Verification items for the finished model (mm, model axes). Face numbers are marked on the shaded views. A direction names the side the tool comes from. Round coordinates to 2 decimals unless told otherwise and drop trailing zeros. Write each loop counter-clockwise with the first axis right and the second up, starting at its lowest first coordinate (ties: lowest second). Pieces come first, ordered by that corner, then holes.
from build123d import *

# Parameters (mm, degrees)
F0_W     = 50.8894138038
F0_H     = 50.8894175291
F1_DEPTH = 50.8
F2_W     = 25.4447069019
F2_H     = 25.3969691694
F3_DEPTH = 50.8
F5_DEPTH = 25.4


with BuildPart() as f1:
    # F0 (on Front) → F1 (new body)
    with BuildSketch(Plane.XZ):
        with Locations((25.4447069019, 25.4447087646)):
            Rectangle(F0_W, F0_H)
    extrude(amount=F1_DEPTH)

    # F2 (on face) → F3 (cut)
    with BuildSketch(Plane.XZ.offset(50.8)):
        with Locations((38.1670603529, 38.1909329444)):
            Rectangle(F2_W, F2_H)
    extrude(amount=-F3_DEPTH, mode=Mode.SUBTRACT)

    # F4 (on face) → F5 (join)
    with BuildSketch(Plane.YZ.offset(25.4447069019)):
        Polygon((0, 50.8894175291), (-25.4, 50.8894175291), (-25.4, 25.4924483597), (0, 25.4924483597), (0, 29.243901372), (0, 43.372977525), align=None)
    extrude(amount=F5_DEPTH)


solid = f1.part
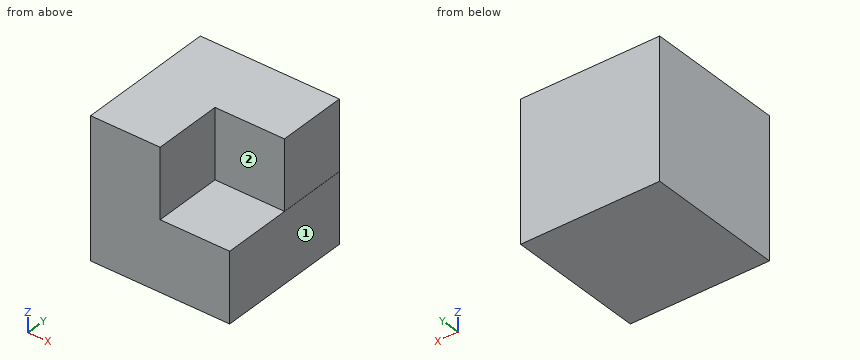
Q1. Sectioned sample at B-B (y = -29). Enter the section's corners in (x, z), plus the area to 3 significant figures.
Recorded:
outline: (0, 0) - (50.89, 0) - (50.89, 25.49) - (25.44, 25.49) - (25.44, 50.89) - (0, 50.89) - close
area: 1,940 mm2
Q2. Material ranges on line 1 along Y through (x, z) = (34, 27); line 2 along Z through (x, y) = (47, -35.5); line 3 along X through (y, z) = (-45, 30), recorded low to high.
Recorded:
line 1: y = -25.4 to 0
line 2: z = 0 to 25.49
line 3: x = 0 to 25.44
Q3. Depth check by flat-ended pin: P1, Ø3, axis at x = 31.5, y = -42.5, coming from the +Z side; P2, Ø7.5, axis at y = -41.5, z = 33, coming from the +X side; P3, Ø7.5, axis at y = -14.5, z = 32.5, coming from the +X side. Enter the tip coordinate at first touch or a pass-through.
Recorded:
P1: stops at z = 25.49
P2: stops at x = 25.44
P3: stops at x = 50.84
Q4. Sectioned sample at A-A (z = 47.5). Enter the section's corners in (x, y).
Recorded:
outline: (0, -50.8) - (25.44, -50.8) - (25.44, -25.4) - (50.84, -25.4) - (50.84, 0) - (0, 0) - close
Q5. Tool access check on the marked faces 1 and 2. Record the directions out of +Z, -Z, +X, -X, +Y, -Y that give a thin tool (end or side, any length) a straight path to the whole face; none if there is none.
Recorded:
face 1: +Z, -Z, +X, +Y, -Y
face 2: +Z, +X, -Y
